Here's how the part is built. I have some questions about the finished solid (model axes, mm). A direction names the side the tool comes from. Round coordinates to 2 decimals unless told otherwise and drop trailing zeros. Order: outer loops, then holes, each group sorted by start corner. A loop starts at its lowest first (then second) coordinate and runs counter-clockwise, first axis right, second up. Notation, with made-up numbers: M -4,77.25 L 52,77.25 A25 ccw 52,114.25 Z; hole C -35.75,51 d5. An arc over 180 degrees is marked long. Write item = value, one per line. Start each with the question number.
Item 1: Please list where these lines run through material, in increasing order: L1, parallel to Z at x = 0, y = 1.6; L2, parallel to X at y = 25, z = 85; L3, parallel to X at y = 58, z = 80.
Item 2: I want a section at C-C, the plane y = 74.5. List the corners of the cut face in (x, z) for me, plus the area to 3 significant figures.
Item 3: I want a section at D-D, the plane x = -59.5. List the corners of the cut face in (y, z) for me, plus the area to 3 significant figures.
Item 4: For faces 1 (the face through (66.91, 51.3, -43.64)), 2 (the face through (3, 0, 7)), which set-ups out of +Z, -Z, +X, -X, +Y, -Y let a thin tool reach every point of the face, with its end or its side?
Item 5: I want a section at B-B, the plane z = 85. List the corners of the cut face in (x, y) for me.
Item 6: We'd pull the mould along X, two halves only. Please class faces 3 (the face through (3, 2, -107)), 4 (the face through (80.1, 51.3, 210.64)), 5 (the face through (2, 2, 87)): pulls with the +X half, pulls with the -X half, needs draft (parallel to the pull), parting line crosses it, or undercut.
Item 7: I want a section at A-A, the plane x = 0. List the corners of the cut face in (y, z) for me.
Item 8: I'm going to push flat-ended pins straight in: P1, Ø5, axis at y = 57.5, z = 116, coming from the -X side; P2, Ø3, axis at x = 30.5, z = 217, coming from the -Y side; P3, Ø10, axis at x = -85.5, y = 78, coming from the +Z side; P4, Ø4, axis at x = -42, y = 12.5, coming from the +Z side. Where does each tip first touch, or does it pass through?
Autodesk Inventor part; units mm, degrees
ref_plane "YZ Plane" through (0, 0, 0) normal (1, 0, 0) x (0, 1, 0)
ref_plane "XZ Plane" through (0, 0, 0) normal (0, 1, 0) x (-1, 0, 0)
ref_plane "XY Plane" through (0, 0, 0) normal (0, 0, 1) x (1, 0, 0)
sketch "Sketch1" plane through (0, 0, 0) normal (0, 1, 0) x (-1, 0, 0)
  line L0 (215, 515) -> (-215, 515)
  line L1 (-215, 515) -> (-215, -515)
  line L2 (-215, -515) -> (215, -515)
  line L3 (215, -515) -> (215, 515)
  line L4 (215, 515) -> (-215, -515) construction
  line L5 (-215, 515) -> (215, -515) construction
  point P0 (0, 0)
  dimension "d0" = 430
  dimension "d1" = 1030
extrude "Plate1" add sketch "Sketch1" along normal blind 2
sketch "Sketch2" plane through (0, 2, 0) normal (0, 1, 0) x (1, 0, 0)
  circle A0 centre (0, -85) radius 145
  line L0 (215, -515) -> (-215, -515)
  circle A1 centre (0, -85) radius 149
  point P0 (0, 0)
  dimension "d3" = 430
  dimension "d4" = 290
  dimension "d5" = 0
  dimension "d6" = 4
extrude "Extrusion1" add sketch "Sketch2" along normal blind 100
sketch "Sketch3" plane through (0, 2, 0) normal (0, 1, 0) x (1, 0, 0)
  circle A0 centre (0, 273.2302) radius 10.795
  point P0 (0, 0)
  dimension "d10" = 21.59
extrude "Cut1" cut sketch "Sketch3" against normal through all
equation "\"d11\" = Thickness"
equation "\"d2\" = Thickness"
equation "\"BendRadius\" = Thickness"
equation "\"BendReliefWidth\" = Thickness"
equation "\"BendReliefDepth\" = 0.5 * Thickness"
equation "\"CornerReliefSize\" = 4 * Thickness"
equation "\"MinimumRemnant\" = 2 * Thickness"
equation "\"TransitionRadius\" = BendRadius"
equation "\"JacobiRadiusSize\" = BendRadius"
equation "\"GapSize\" = Thickness"
properties part number "mid Base"
Filled in:
q1.L1 = -515 to -284.03, -262.44 to 515
q1.L2 = -149 to -145, 145 to 149
q1.L3 = -148.92 to -144.91, 144.91 to 148.92
q2.outline = C 0,85 d298; hole C 0,85 d290
q2.area = 3,690 mm^2
q3.outline = M 0,-515 L 2,-515 L 2,-51.6 L 102,-51.6 L 102,-47.23 L 2,-47.23 L 2,217.23 L 102,217.23 L 102,221.6 L 2,221.6 L 2,515 L 0,515 Z
q3.area = 2,930 mm^2
q4.face_1 = +Y
q4.face_2 = +Z, -Z, +X, -X, -Y
q5.outline = M -215,0 L 215,0 L 215,2 L 149,2 L 149,102 L 145,102 L 145,2 L -145,2 L -145,102 L -149,102 L -149,2 L -215,2 Z
q6.face_3 = needs draft
q6.face_4 = parting line crosses it
q6.face_5 = undercut
q7.outline = M 0,-515 L 2,-515 L 2,-284.03 L 0,-284.03 Z; M 0,-262.44 L 2,-262.44 L 2,-64 L 102,-64 L 102,-60 L 2,-60 L 2,230 L 102,230 L 102,234 L 2,234 L 2,515 L 0,515 Z
q8.P1 = -146.25
q8.P2 = 0
q8.P3 = 210.38
q8.P4 = 228.53
